from build123d import *

# Parameters (mm, degrees)
SKETCH3_W           = 4.7625
SKETCH3_H           = 3.175
SKETCH3_W_2         = 3.175
SKETCH3_H_2         = 6.35
BOSS_EXTRUDE2_DEPTH = 3.175


with BuildPart() as part:
    # Sketch3 → Boss-Extrude2 (new body)
    with BuildSketch(Plane(origin=(0, 88.979885655, 2.951534319), x_dir=(1, 0, 0), z_dir=(0, 0.9994503024750413, 0.03315256977292581))):
        Polygon((73.130884883, -481.824366224), (73.130884883, -469.124366224), (-15.769115117, -469.124366224), (-15.769115117, -481.824366224), (-12.594115117, -481.824366224), (-12.594115117, -507.224366224), (-15.769115117, -507.224366224), (-15.769115117, -519.924366224), (73.130884883, -519.924366224), (73.130884883, -507.224366224), (69.955884883, -507.224366224), (69.955884883, -481.824366224), align=None)
        with Locations((28.684303559, -483.221366224)):
            Rectangle(SKETCH3_W, SKETCH3_H, mode=Mode.SUBTRACT)
        with Locations((28.680884883, -507.426337868)):
            Rectangle(SKETCH3_W_2, SKETCH3_H_2, mode=Mode.SUBTRACT)
        with BuildLine():
            Line((13.62075844, -483.734366224), (3.12075844, -483.734366224))
            ThreePointArc((3.12075844, -483.734366224), (2.519717676, -483.98332546), (2.27075844, -484.584366224))
            Line((2.27075844, -484.584366224), (2.27075844, -505.384366224))
            ThreePointArc((2.27075844, -505.384366224), (2.519717676, -505.985406988), (3.12075844, -506.234366224))
            Line((3.12075844, -506.234366224), (13.62075844, -506.234366224))
            ThreePointArc((13.62075844, -506.234366224), (14.221799204, -505.985406988), (14.47075844, -505.384366224))
            Line((14.47075844, -505.384366224), (14.47075844, -484.584366224))
            ThreePointArc((14.47075844, -484.584366224), (14.221799204, -483.98332546), (13.62075844, -483.734366224))
        make_face(mode=Mode.SUBTRACT)
        with BuildLine():
            ThreePointArc((9.350271075, -508.884366224), (9.063378466, -508.191746198), (8.37075844, -507.904853589))
            ThreePointArc((8.37075844, -507.904853589), (7.678138413, -508.191746198), (7.391245805, -508.884366224))
            ThreePointArc((7.391245805, -508.884366224), (7.678138413, -509.576986251), (8.37075844, -509.863878859))
            ThreePointArc((8.37075844, -509.863878859), (9.063378466, -509.576986251), (9.350271075, -508.884366224))
        make_face(mode=Mode.SUBTRACT)
        with BuildLine():
            ThreePointArc((8.37075844, -482.084366224), (9.077865221, -481.791473005), (9.37075844, -481.084366224))
            ThreePointArc((9.37075844, -481.084366224), (9.077865221, -480.377259443), (8.37075844, -480.084366224))
            ThreePointArc((8.37075844, -480.084366224), (7.663651658, -480.377259443), (7.37075844, -481.084366224))
            ThreePointArc((7.37075844, -481.084366224), (7.663651658, -481.791473005), (8.37075844, -482.084366224))
        make_face(mode=Mode.SUBTRACT)
    extrude(amount=BOSS_EXTRUDE2_DEPTH)


solid = part.part
Can you work these out from the model? Positions are in its coordinate system, mm. A direction names the side the tool comes from. Give positions to 0.01 mm unless a question says otherwise; leave off trailing zeros. Order: outer loops, then holes, each group sorted by start corner. A loop starts at its lowest first (then second) coordinate and runs counter-clockwise, first axis right, second up. Notation, with made-up numbers: M 10.5,-36.5 L 19.5,-36.5 A20 ccw 19.5,-19.5 Z; hole C 19.5,-14.75 d6. An arc over 180 degrees is marked long. Use one line per item in the form item = value.
Item 1: Will these pins go through, and if not, where does the flat tip stop? pin 1 Ø5 at (x, z) = (15.5, 503.5) entering from +Y; pin 2 Ø5 at (x, z) = (29, 501) entering from +Y; pin 3 Ø2.5 at (y, z) = (74.5, 486.5) entering from -X.
Values follow:
pin_1 = 75.64
pin_2 = 75.72
pin_3 = -12.59
Item 2: If we section it at D-D, the plane z = 475: Write out the boundary of the cut face in (x, y), and give its area (3 significant figures).
Values follow:
outline = M -15.77,73.32 L 73.13,73.32 L 73.13,76.5 L -15.77,76.5 Z
area = 282 mm^2
Item 3: If I drill on line 1 along X through (y, z) = (72.9, 508); line 2 along X through (y, z) = (75.3, 487); line 3 along Y through (x, z) = (16.5, 509), over which ranges is the centre line in solid material (lowest first)? Write a range as [from, to].
Values follow:
line_1 = [-12.59, 2.27], [14.47, 27.09], [30.27, 69.96]
line_2 = [-12.59, 2.35], [14.4, 26.3], [31.07, 69.96]
line_3 = [72.19, 75.37]
Item 4: If we section it at A-A, the plane x = 29: Write out the boundary of the cut face in (y, z).
Values follow:
outline = M 71.74,522.59 L 72.05,513.27 L 75.23,513.38 L 74.92,522.7 Z; M 72.26,506.93 L 72.91,487.49 L 76.08,487.6 L 75.44,507.03 Z; M 73.01,484.32 L 73.43,471.82 L 76.6,471.92 L 76.19,484.43 Z
Item 5: For faces 4 (the flat face through (73.131, 74, 516)), 5 (the flat face through (69.956, 74, 497)), which set-ups out of +Z, -Z, +X, -X, +Y, -Y let a thin tool reach every point of the face, with its end or its side?
Values follow:
face_4 = +Z, -Z, +X, +Y, -Y
face_5 = +X, +Y, -Y
Item 6: Thinking about a two-plate mould opening in X: for faces 1 (the flat face through (73.131, 75, 478)), 2 (the flat face through (31.066, 75, 486)), 3 (the flat face through (-15.769, 74, 516)), which applies, pulls with the +X half, pulls with the -X half, needs draft (parallel to the pull), parting line crosses it, or undercut?
Values follow:
face_1 = pulls with the +X half
face_2 = undercut
face_3 = pulls with the -X half
Item 7: If we section it at C-C, the plane x = 64: Write out the boundary of the cut face in (y, z), and give its area (3 significant figures).
Values follow:
outline = M 71.74,522.59 L 73.43,471.82 L 76.6,471.92 L 74.92,522.7 Z
area = 161 mm^2
Item 8: If we section it at B-B, the plane z = 497: Write out the boundary of the cut face in (x, y), and give its area (3 significant figures).
Values follow:
outline = M -12.59,72.59 L 2.27,72.59 L 2.27,75.77 L -12.59,75.77 Z; M 14.47,72.59 L 69.96,72.59 L 69.96,75.77 L 14.47,75.77 Z
area = 223 mm^2
